Here's how the part is built. I have some questions about the finished solid (model axes, mm). A direction names the side the tool comes from. Give positions to 0.01 mm unless a question says otherwise; leave off trailing zeros. Write each loop counter-clockwise with the first axis right and the second up, starting at its lowest first coordinate (ties: lowest second). Pieces come first, ordered by that corner, then holes. Notation, with made-up numbers: (14, 52) - (27, 52) arc R4 cw to (27, 57) - close; hole circle Ø7 at (18.25, -34). An arc over 180 degrees is marked (long way). One line per item, written item: value. Start each with the question number.
1) I'm going to push a flat-ended pin straight in: P1, Ø2, axis at x = 2, z = 29.5, coming from the -Y side. Where does the tip first touch, or does it pass through?
2) Please list where these lines run through material, in increasing order: L1, parallel to X at y = -226.5, z = 16; L2, parallel to Y at x = -11, z = 34.5; L3, parallel to Z at x = -129, y = 126. Write a range as [from, to].
3) On a 3-axis mill with a long thin cutter (end or side, diameter ignored), from which of +Z, -Z, +X, -X, +Y, -Y can I reach the whole of each face in a straight line? I mean faces 5 (the flat face through (-1, 246, 38.1)), 6 (the flat face through (241.3, -9, 25)). Say none if no direction works.
4) We'd pull the mould along X, two halves only. Please class faces 1 (the flat face through (266.7, -4, 19)), 2 (the flat face through (-3, -9, 12.7)), 3 (the flat face through (4, 254, 19)), 4 (the flat face through (-266.7, 4, 19)): +X half, -X half, draft (parallel to the pull), parting line (faces both ways), or undercut.
5) Imagine slicing it at A-A on z = 22.5. Write out the boundary of the cut face in (x, y), plus the area to 3 significant figures.
6) Imagine slicing it at B-B on y = 94.5. Write out the boundary of the cut face in (x, z), plus the area to 3 significant figures.
7) Imagine slicing it at C-C on x = 225. Write out the boundary of the cut face in (y, z).
from build123d import *

# Parameters (mm, degrees)
F1_DEPTH = 12.7
F2_W     = 482.6
F2_H     = 25.4
F3_DEPTH = 25.4


with BuildPart() as f1:
    # F0 (on Top) → F1 (new body)
    with BuildSketch(Plane.XY):
        Polygon((-241.3, 254), (-266.7, 254), (-266.7, -254), (266.7, -254), (266.7, 254), (241.3, 254), align=None)
    extrude(amount=F1_DEPTH)

    # F2 (on face) → F3 (join)
    with BuildSketch(Plane.XY.offset(12.7)):
        with Locations((0, 241.3)):
            Rectangle(F2_W, F2_H)
        Polygon((-241.3, 254), (-266.7, 254), (-266.7, -254), (-241.3, -254), (-241.3, 228.6), align=None)
        Polygon((266.7, 254), (241.3, 254), (241.3, 228.6), (241.3, -254), (266.7, -254), align=None)
    extrude(amount=F3_DEPTH)


solid = f1.part
Numbers:
1. P1: y = 228.6
2. L1: [-266.7, -241.3], [241.3, 266.7]
2. L2: [228.6, 254]
2. L3: [0, 12.7]
3. face 5: +Z, +X, -X, +Y, -Y
3. face 6: +Z, -Y
4. face 1: +X half
4. face 2: undercut
4. face 3: draft
4. face 4: -X half
5. outline: (-266.7, -254) - (-241.3, -254) - (-241.3, 228.6) - (241.3, 228.6) - (241.3, -254) - (266.7, -254) - (266.7, 254) - (-266.7, 254) - close
5. area: 38,100 mm^2
6. outline: (-266.7, 0) - (266.7, 0) - (266.7, 38.1) - (241.3, 38.1) - (241.3, 12.7) - (-241.3, 12.7) - (-241.3, 38.1) - (-266.7, 38.1) - close
6. area: 8,060 mm^2
7. outline: (-254, 0) - (254, 0) - (254, 38.1) - (228.6, 38.1) - (228.6, 12.7) - (-254, 12.7) - close
